Geometry: see drawing. Coordinates: mm, zero at the bounding-box minimum. A direction names the side the tool comes from. Round coordinates to 2 decimals unless told otherwise and drop trailing zeros. Order: outer loops, then holes, each group sorted by start corner. A loop starts at its lowest first (then second) coordinate and runs counter-clockwise, first axis right, second up. Notation, with made-up numbers: (11, -31.5) -> (61, -31.5) arc R19 ccw to (61, -7.5) -> close; hole circle Ø4 at (44, 37.5). An arc over 180 degrees is marked (long way). Write item = value, one per line. Start each with the question number.
(1) Ray query, line 1 (Y direction, x = 1.5, z = 3); line 2 (Z direction, x = 6.25, y = 6.5); line 3 (X direction, y = 2, z = 2). Return the intervals inside material, ascending.
(2) Cut plane B-B on x = 3.75. Return the cut outline in (y, z).
(3) Cut plane D-D on z = 8.25. Return the cut outline in (x, y).
(4) Cut plane A-A on y = 3.75. Return the cut outline in (x, z).
(5) Contact query for flat-ended pins moving along their axis: pin 1 Ø3.5 at (y, z) = (4, 5.5) entering from -X; pin 2 Ø0.7 at (x, y) = (3, 6.5) entering from -Z; pin 3 Ø2 at (y, z) = (2, 2) entering from +X. Output: stop coordinate, or through.
(6) Reachability of the marked faces 1, 2, 3 and 4 from +Z, -Z, +X, -X, +Y, -Y: full face, straight path, thin tool, end or side. Return the list, or none.
(7) Cut plane C-C on z = 6.25. Return the cut outline in (x, y).
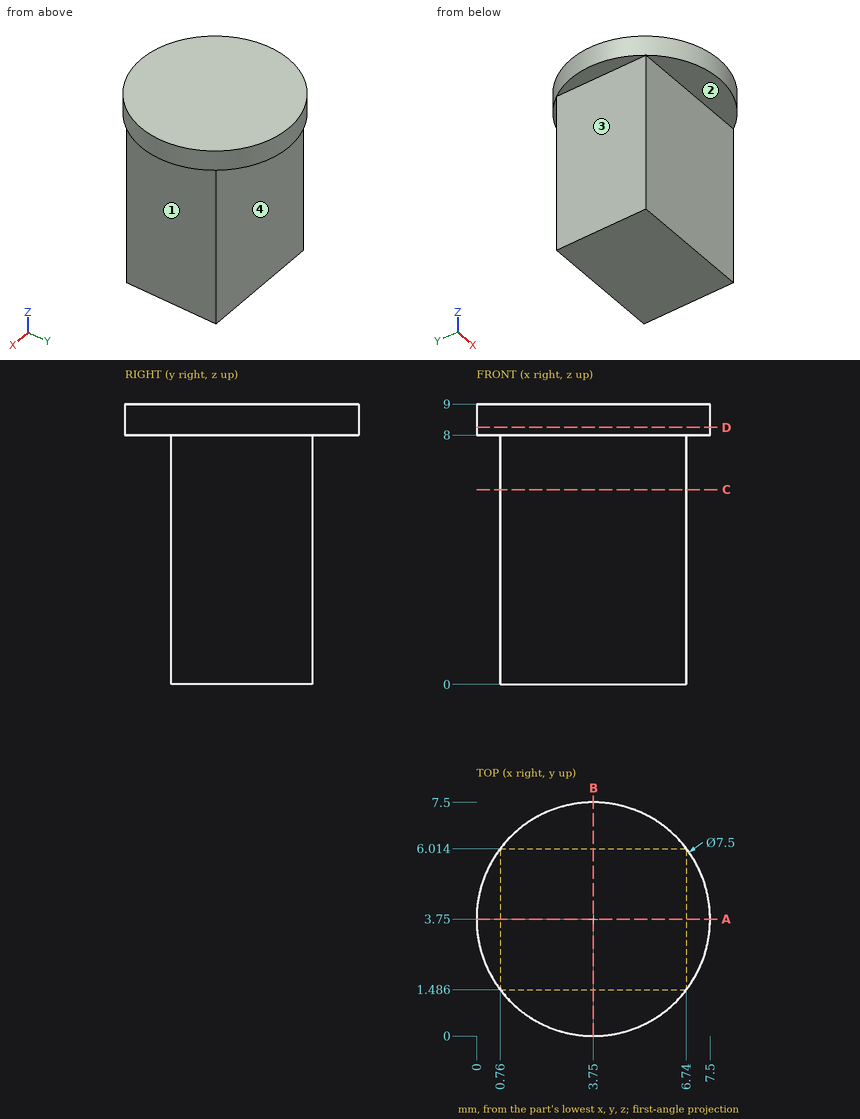
Evaluation:
q1.line_1 = 1.49 to 6.01
q1.line_2 = 8 to 9
q1.line_3 = 0.76 to 6.74
q2.outline = (0, 8) -> (1.49, 8) -> (1.49, 0) -> (6.01, 0) -> (6.01, 8) -> (7.5, 8) -> (7.5, 9) -> (0, 9) -> close
q3.outline = circle Ø7.5 at (3.75, 3.75)
q4.outline = (0, 8) -> (0.76, 8) -> (0.76, 0) -> (6.74, 0) -> (6.74, 8) -> (7.5, 8) -> (7.5, 9) -> (0, 9) -> close
q5.pin_1 = 0.76
q5.pin_2 = 8
q5.pin_3 = 6.74
q6.face_1 = -Z, +X, +Y, -Y
q6.face_2 = -Z, +X, -X, -Y
q6.face_3 = -Z, -X, +Y, -Y
q6.face_4 = -Z, +X, -X, +Y
q7.outline = (0.76, 1.49) -> (6.74, 1.49) -> (6.74, 6.01) -> (0.76, 6.01) -> close
